The figure shows three views and two pictorial views of one solid part (mm, origin at its lowest corner). Answer the questions. A direction names the side the tool comes from. Give positions to 0.01 mm unless a question says otherwise; leave off trailing zeros. Loops run counter-clockwise (first coordinate to the right, second up) from the corner with the lowest first, then second, coordinate; pieces in that order, holes last. Notation, with made-up numbers: (72.25, -22) - (104.25, -22) arc R14 ccw to (104.25, -16) - close; hole circle Ø3 at (81.25, 36). An arc over 180 degrees is marked (long way). Use a Markdown table: item, result. Add a question column.
Item 1: A cutting plane is placed at C-C (x = 19). Determine the outline of the cut face in (y, z).
Item 2: For a pull along Z with two mould halves and no side action, classify the marked faces 1, 2 and 3 as +Z half, -Z half, draft (parallel to the pull), parting line (faces both ways), or undercut.
Item 3: A cutting plane is placed at A-A (z = 40). Determine the outline of the cut face in (x, y), plus the area to 3 significant figures.
Item 4: Which of the six approach directions +Z, -Z, +X, -X, +Y, -Y give full straight-line access (tool end or side, diameter ignored) to the marked faces 4, 5, 6 and 7?
Item 5: A cutting plane is placed at D-D (z = 8). Determine the outline of the cut face in (x, y).
Item 6: A cutting plane is placed at B-B (y = 27). Determine the outline of the cut face in (x, z), plus the area to 3 significant figures.
Item 7: Consider probe 1 along Y at (x, z) = (1.5, 40); probe 2 along Y at (x, z) = (17, 2.6); probe 3 along Z at (x, y) = (20.25, 24.5). Determine where each line is inside the solid, lowest interval first. Write a range as [from, to].
Item 8: Each of these flat-tipped pins is pushed along its axis until it touches: P1, Ø1.5, axis at x = 25, y = 26.5, coming from the +Z side; P2, Ø2.5, axis at y = 33.95, z = 61.4, coming from the +X side; P3, Ø6.5, axis at x = 18.5, z = 5.5, coming from the -Y side; P4, Ø4.5, axis at y = 8.8, z = 53.23, coming from the +X side. Where does it stop, or does it pass through?
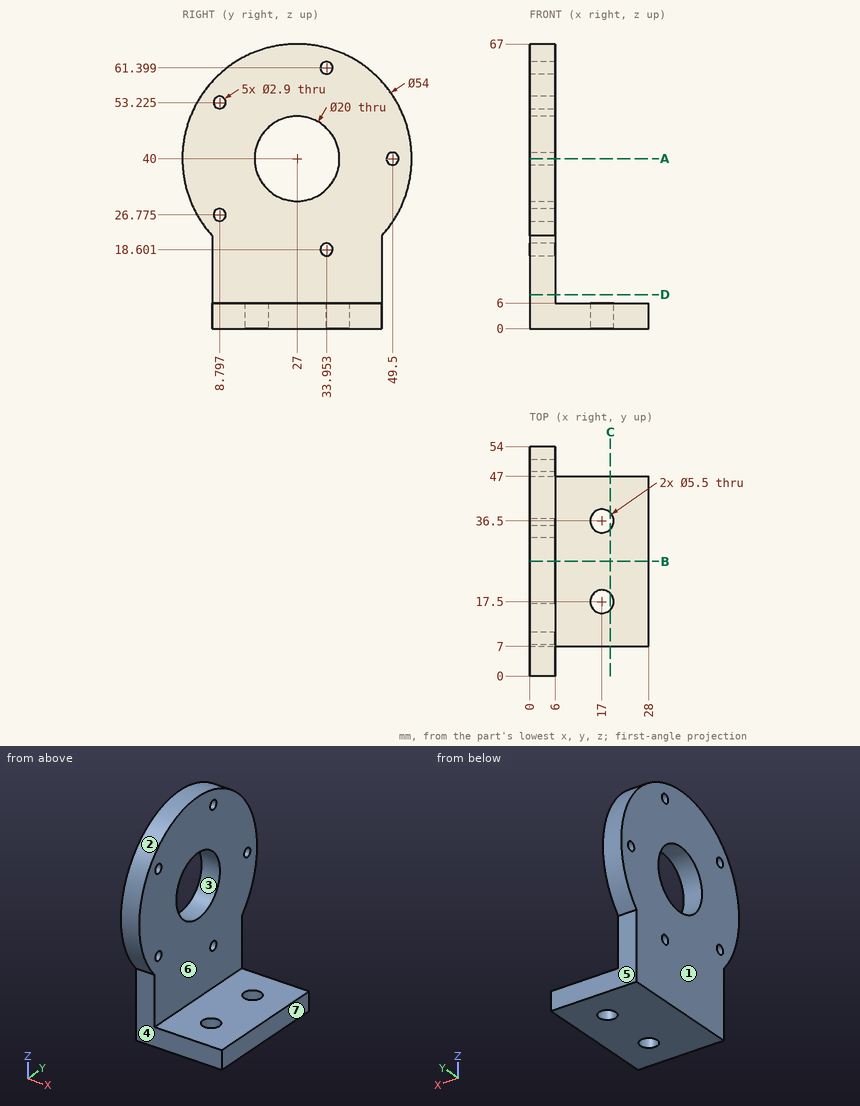
Geometry says:
| question | item | result |
|---|---|---|
| 1 | outline | (7, 0) - (15.61, 0) - (15.61, 6) - (7, 6) - close; (19.39, 0) - (34.61, 0) - (34.61, 6) - (19.39, 6) - close; (38.39, 0) - (47, 0) - (47, 6) - (38.39, 6) - close |
| 2 | face 1 | draft |
| 2 | face 2 | parting line |
| 2 | face 3 | undercut |
| 3 | outline | (0, 0) - (6, 0) - (6, 17) - (0, 17) - close; (0, 37) - (6, 37) - (6, 48.05) - (0, 48.05) - close; (0, 50.95) - (6, 50.95) - (6, 54) - (0, 54) - close |
| 3 | area | 187 mm² |
| 4 | face 4 | -Z, +X, -X, -Y |
| 4 | face 5 | -Z, +X, -X, +Y |
| 4 | face 6 | +Z, +X, +Y, -Y |
| 4 | face 7 | +Z, -Z, +X, +Y, -Y |
| 5 | outline | (0, 7) - (6, 7) - (6, 47) - (0, 47) - close |
| 6 | outline | (0, 0) - (28, 0) - (28, 6) - (6, 6) - (6, 30) - (0, 30) - close; (0, 50) - (6, 50) - (6, 67) - (0, 67) - close |
| 6 | area | 414 mm² |
| 7 | probe 1 | [0, 17], [37, 48.05], [50.95, 54] |
| 7 | probe 2 | [7, 14.75], [20.25, 33.75], [39.25, 47] |
| 7 | probe 3 | [0, 6] |
| 8 | P1 | z = 6 |
| 8 | P2 | through |
| 8 | P3 | y = 7 |
| 8 | P4 | x = 6 |
